Model file for the job. Use its own axes, mm. A direction names the side the tool comes from. Coordinates: 2 decimals unless noted, no trailing zeros. Order: outer loops, then holes, each group sorted by start corner. A loop starts at its lowest first (then second) coordinate and runs counter-clockwise, first axis right, second up. Notation, with made-up numbers: (71, 38) -> (95, 38) arc R24 cw to (95, 70) -> close; hole circle Ø11 at (59.25, 50.5). An arc over 180 degrees is marked (long way). Return JSON: item names as keys, results as strings. Group by question number.
1) Cut at C-C (z = -7). Write the cut outline in (x, y).
2) Which spindle directions (+Z, -Z, +X, -X, +Y, -Y) get a long thin tool onto all of the face, cutting with end or side? Do faces 1 (the flat face through (-76.2, 2, 9)), 2 (the flat face through (-76.2, 2, -9)), 3 (the flat face through (76.2, 2, -9)), 4 (the flat face through (76.2, 2, 9)). Say none if no direction does.
3) Pull direction Z, two halves, no side cores. Call faces 5 (the cylindrical face through (-75.773, 1.612, -0.478)), 6 (the cylindrical face through (78.8, 1.6, -0.5)), 7 (the flat face through (-1, 3.18, 0)), 8 (the flat face through (78, 2, -5)): +Z half, -Z half, draft (parallel to the pull), parting line (faces both ways), or undercut.
4) Flat gauge pins, fed straight in: pin 1 (1.6 mm diameter, centred on x = -77.5, y = 1.5, fed in from +Z); pin 2 (1 mm diameter, centred on y = 1.5, z = -7, fed in from +X); pin 3 (1 mm diameter, centred on y = 2, z = -9.5, fed in from -X). Where does each tip first touch, or does it go through?
5) Cut at A-A (y = 2.1). Write the cut outline in (x, z).
6) Cut at B-B (z = 0). Write the cut outline in (x, y), and give its area (3 significant figures).
7) Probe line 1 (X direction, y = 1.55, z = 0); line 2 (Z direction, x = -77.29, y = 1.4); line 3 (X direction, y = 2.6, z = 0.5). List the from-to ranges inside material, lowest first.
from build123d import *

# Parameters (mm, degrees)
SKETCH2_W           = 152.4
SKETCH2_H           = 25.4
BOSS_EXTRUDE1_DEPTH = 3.18
SKETCH3_W           = 10
SKETCH3_H           = 3.18
BOSS_EXTRUDE2_DEPTH = 3.18
SKETCH4_W           = 10
SKETCH4_H           = 3.18
BOSS_EXTRUDE3_DEPTH = 3.18
SKETCH5_R           = 1.59
CUT_EXTRUDE1_DEPTH  = 3.18


with BuildPart() as part:
    # Sketch2 → Boss-Extrude1 (new body)
    with BuildSketch(Plane(origin=(0, 0, 0), x_dir=(1, 0, 0), z_dir=(0, 1, 0))):
        Rectangle(SKETCH2_W, SKETCH2_H)
    extrude(amount=BOSS_EXTRUDE1_DEPTH)

    # Sketch3 → Boss-Extrude2 (add)
    with BuildSketch(Plane.ZY.offset(76.2)):
        with Locations((0, 1.59)):
            Rectangle(SKETCH3_W, SKETCH3_H)
    extrude(amount=BOSS_EXTRUDE2_DEPTH)

    # Sketch4 → Boss-Extrude3 (add)
    with BuildSketch(Plane(origin=(76.2, 0, 0), x_dir=(0, 0, -1), z_dir=(1, 0, 0))):
        with Locations((0, 1.59)):
            Rectangle(SKETCH4_W, SKETCH4_H)
    extrude(amount=BOSS_EXTRUDE3_DEPTH)

    # Sketch5 → Cut-Extrude1 (cut)
    with BuildSketch(Plane(origin=(0, 3.18, 0), x_dir=(1, 0, 0), z_dir=(0, 1, 0))):
        with Locations((77.29, 0)):
            Circle(SKETCH5_R)
        with Locations((-77.29, 0)):
            Circle(SKETCH5_R)
    extrude(amount=-CUT_EXTRUDE1_DEPTH, mode=Mode.SUBTRACT)


solid = part.part
Answers below:
{
 "1": {"outline": "(-76.2, 0) -> (76.2, 0) -> (76.2, 3.18) -> (-76.2, 3.18) -> close"},
 "2": {"face 1": "+Z, -X, +Y, -Y", "face 2": "-Z, -X, +Y, -Y", "face 3": "-Z, +X, +Y, -Y", "face 4": "+Z, +X, +Y, -Y"},
 "3": {"face 5": "undercut", "face 6": "undercut", "face 7": "draft", "face 8": "-Z half"},
 "4": {"pin 1": "stops at z = 5", "pin 2": "stops at x = 76.2", "pin 3": "stops at x = -76.2"},
 "5": {"outline": "(-79.38, -5) -> (-76.2, -5) -> (-76.2, -12.7) -> (76.2, -12.7) -> (76.2, -5) -> (79.38, -5) -> (79.38, 5) -> (76.2, 5) -> (76.2, 12.7) -> (-76.2, 12.7) -> (-76.2, 5) -> (-79.38, 5) -> close; hole circle Ø3.18 at (-77.29, 0); hole circle Ø3.18 at (77.29, 0)"},
 "6": {"outline": "(-79.38, 0) -> (-78.88, 0) -> (-78.88, 3.18) -> (-79.38, 3.18) -> close; (-75.7, 0) -> (75.7, 0) -> (75.7, 3.18) -> (-75.7, 3.18) -> close; (78.88, 0) -> (79.38, 0) -> (79.38, 3.18) -> (78.88, 3.18) -> close", "area": "485 mm^2"},
 "7": {"line 1": "x = -79.38 to -78.88, -75.7 to 75.7, 78.88 to 79.38", "line 2": "z = -5 to -1.59, 1.59 to 5", "line 3": "x = -79.38 to -78.8, -75.78 to 75.78, 78.8 to 79.38"}
}
